Verification items for the finished model (mm, model axes). A direction names the side the tool comes from. Round coordinates to 2 decimals unless told otherwise and drop trailing zeros. Write each loop counter-clockwise with the first axis right and the second up, starting at its lowest first coordinate (ties: lowest second). Pieces come first, ordered by that corner, then holes. Notation, with made-up numbers: M 85,85.25 L 94,85.25 A16 ccw 94,99.25 Z; hole C 60.5,43 d5. An arc over 180 degrees is marked long. One line per question, with ' | ' between items. Start each with the question number.
Q1. Tool access check on faces 1 (the face through (0, 0, 21)), 2 (the face through (0, 2, 1)). Record the directions out of +Z, -Z, +X, -X, +Y, -Y that give a thin tool (end or side, any length) a straight path to the whole face; none if there is none.
Q2. Cross-section at C-C (y = -1.25). Record the boundary of the cut face in (x, z), then the cut area to 3 significant figures.
Q3. Thickness scan on line 1 along Z through (x, y) = (3.5, -0.5); line 2 along X through (y, z) = (3.75, 4.5); line 3 along Z through (x, y) = (1.5, 0). Record the ranges inside material, lowest first. Write a range as from..to.
Q4. Cross-section at A-A (z = 2.5). Record the boundary of the cut face in (x, y).
Q5. Release check for a two-part mould opening along X. For faces 3 (the face through (-0.54, 2.44, 12.89)), 4 (the face through (0, -2, 1)), 5 (the face through (2, -2, 5)) record: released by +X, released by -X, zero draft, split by the parting line, or undercut.
Q6. Cross-section at B-B (x = 0). Record the boundary of the cut face in (y, z), then the cut area to 4 significant figures.
Q7. Cross-section at D-D (z = 14.75). Record the boundary of the cut face in (x, y), then the cut area to 3 significant figures.
Q8. Gauge pin test, flat ends, axial feed: pin 1 (2 mm diameter, centred on y = -1.5, z = 3.5, fed in from -X); pin 2 (4 mm diameter, centred on x = 1.5, y = 1, fed in from -Z). Record the tip position at first contact, or that the pin passes through.
Autodesk Inventor part; units mm, degrees
ref_plane "YZ Plane" through (0, 0, 0) normal (1, 0, 0) x (0, 1, 0)
ref_plane "XZ Plane" through (0, 0, 0) normal (0, 1, 0) x (-1, 0, 0)
ref_plane "XY Plane" through (0, 0, 0) normal (0, 0, 1) x (1, 0, 0)
sketch "Sketch1" plane through (0, 0, 0) normal (0, 0, 1) x (1, 0, 0)
  circle A0 centre (0, 0) radius 4.25
  dimension "d0" = 8.5
extrude "Extrusion1" add sketch "Sketch1" along normal blind 5
sketch "Sketch2" plane through (0, 0, 5) normal (0, 0, 1) x (1, 0, 0)
  circle A0 centre (0, 0) radius 4.25
  circle A1 centre (0, 0) radius 2.5
  dimension "d3" = 5
extrude "Extrusion2" add sketch "Sketch2" along normal blind 16 contours A1
sketch "Sketch3" plane through (0, 0, 0) normal (0, 0, -1) x (-1, 0, 0)
  circle A0 centre (0, 0) radius 4.25
  line L0 (2.3094, 0) -> (1.1547, -2)
  line L1 (1.1547, -2) -> (-1.1547, -2)
  line L2 (-1.1547, -2) -> (-2.3094, 0)
  line L3 (-2.3094, 0) -> (-1.1547, 2)
  line L4 (-1.1547, 2) -> (1.1547, 2)
  line L5 (1.1547, 2) -> (2.3094, 0)
  dimension "d6" = 4
extrude "Extrusion3" cut sketch "Sketch3" against normal blind 3 contours L0 L1 L2 L3 L4 L5
thread "Thread1"
properties part number "m5x1"
Determined:
1) face 1: +Z, +X, -X, +Y, -Y | face 2: -Z
2) outline: M -4.06,0 L -1.59,0 L -1.59,3 L 1.59,3 L 1.59,0 L 4.06,0 L 4.06,5 L 2.17,5 L 2.17,21 L -2.17,21 L -2.17,5 L -4.06,5 Z | area: 100 mm²
3) line 1: z = 0..5 | line 2: x = -2..2 | line 3: z = 3..21
4) outline: C 0,0 d8.5; hole M -2.31,0 L -1.15,-2 L 1.15,-2 L 2.31,0 L 1.15,2 L -1.15,2 Z
5) face 3: split by the parting line | face 4: undercut | face 5: zero draft
6) outline: M -4.25,0 L -2,0 L -2,3 L 2,3 L 2,0 L 4.25,0 L 4.25,5 L 2.5,5 L 2.5,21 L -2.5,21 L -2.5,5 L -4.25,5 Z | area: 110.5 mm²
7) outline: C 0,0 d5 | area: 19.6 mm²
8) pin 1: stops at x = -4.22 | pin 2: stops at z = 0
